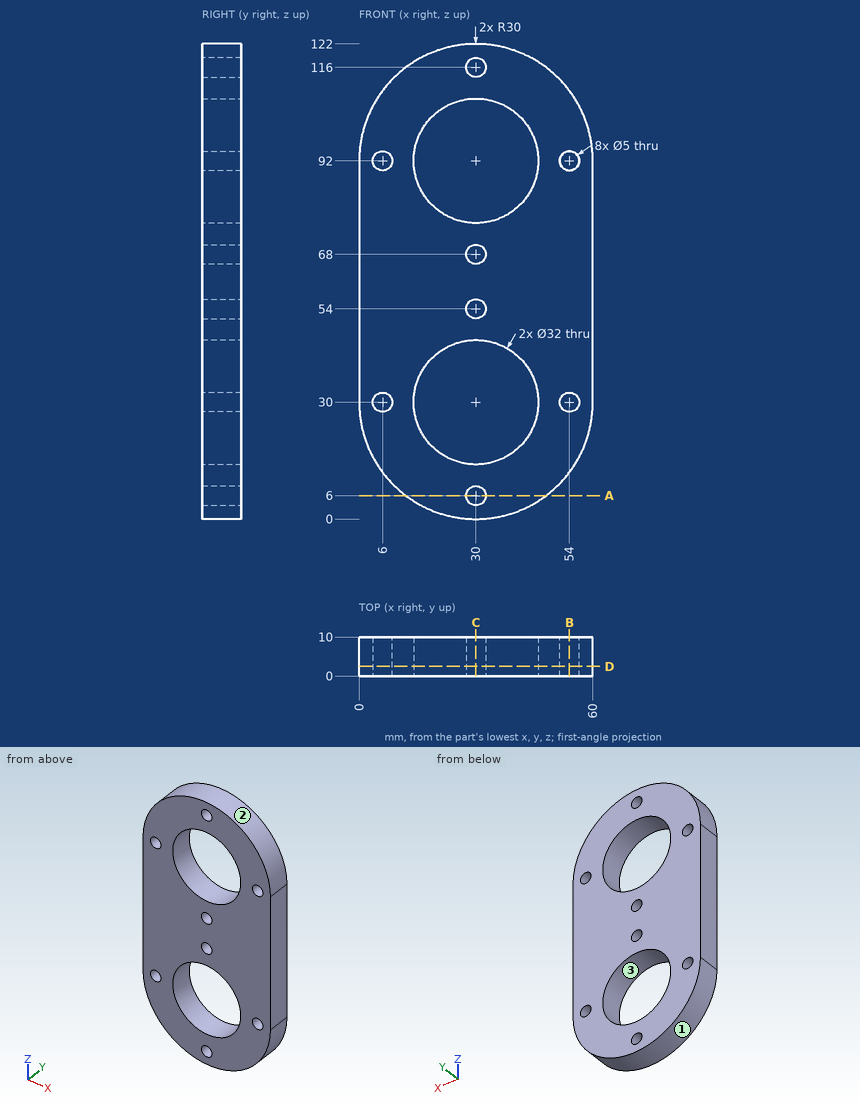
Design review of the part shown in the three views and the two pictorial views. Dimensions are in mm from the part's minimum x, y and z. Round coordinates to 2 decimals unless told otherwise and drop trailing zeros. Loops run counter-clockwise (first coordinate to the right, second up) from the corner with the lowest first, then second, coordinate; pieces in that order, holes last.
Q1. Add section D-D on y = 2.5. Give the number of separate pieces and of enclosed holes in the cut face, plus the area to 3 significant figures.
Result sheet:
separate pieces: 1
enclosed holes: 10
area: 4,780 mm2
Q2. Add section A-A on z = 6. Write out the cut boundary in (x, y).
Result sheet:
outline: (12, 0) - (27.5, 0) - (27.5, 10) - (12, 10) - close; (32.5, 0) - (48, 0) - (48, 10) - (32.5, 10) - close
Q3. Mouldability with a two-part tool opening along Z and no side actions: class the marked faces 1, 2 and 3 as +Z half, -Z half, draft (parallel to the pull), parting line (faces both ways), or undercut.
Result sheet:
face 1: -Z half
face 2: +Z half
face 3: undercut
Q4. Add section B-B on x = 54. Write out the cut boundary in (y, z).
Result sheet:
outline: (0, 12) - (10, 12) - (10, 27.5) - (0, 27.5) - close; (0, 32.5) - (10, 32.5) - (10, 89.5) - (0, 89.5) - close; (0, 94.5) - (10, 94.5) - (10, 110) - (0, 110) - close
Q5. Insertion check: pin 1 Ø1.5 at (y, z) = (6.5, 17.5) entering from -X; pin 2 Ø2 at (y, z) = (5, 24.5) entering from +X; pin 3 Ø1 at (x, y) = (12, 3.5) entering from +Z. Each pin has a flat end and moves straight along its axis. Give the tip position at first contact, or say it passes through.
Result sheet:
pin 1: stops at x = 2.4
pin 2: stops at x = 59.66
pin 3: stops at z = 116.37
Q6. Add section C-C on x = 30. Write out the cut boundary in (y, z).
Result sheet:
outline: (0, 0) - (10, 0) - (10, 3.5) - (0, 3.5) - close; (0, 8.5) - (10, 8.5) - (10, 14) - (0, 14) - close; (0, 46) - (10, 46) - (10, 51.5) - (0, 51.5) - close; (0, 56.5) - (10, 56.5) - (10, 65.5) - (0, 65.5) - close; (0, 70.5) - (10, 70.5) - (10, 76) - (0, 76) - close; (0, 108) - (10, 108) - (10, 113.5) - (0, 113.5) - close; (0, 118.5) - (10, 118.5) - (10, 122) - (0, 122) - close
Q7. To check wall thickness, follow line 1 along Z through (x, y) = (35.5, 6.5); line 2 along Z through (x, y) = (7, 8.75); line 3 along X through (y, z) = (1.25, 96). State the ranges of each line that lie inside material, in increasing order.
Result sheet:
line 1: z = 0.51 to 14.98, 45.02 to 76.98, 107.02 to 121.49
line 2: z = 10.74 to 27.71, 32.29 to 89.71, 94.29 to 111.26
line 3: x = 0.27 to 14.51, 45.49 to 59.73
